```python
from build123d import *

# Parameters (mm, degrees)
F1_DEPTH = 50.8
F2_W     = 25.4
F2_H     = 15.645319
F3_DEPTH = 50.8
F4_W     = 21.66615
F4_H     = 13.618723
F5_DEPTH = 85.344


with BuildPart() as f1:
    # F0 (on Front) → F1 (new body)
    with BuildSketch(Plane.XZ):
        with BuildLine():
            Line((12.7, 38.1), (0, 38.1))
            Line((0, 38.1), (0, 0))
            Line((0, 0), (31.75, 0))
            Line((31.75, 0), (31.75, 12.7))
            ThreePointArc((31.75, 12.7), (19.301518, 23.207389), (12.7, 38.1))
        make_face()
    extrude(amount=F1_DEPTH)

    # F2 (on Right) → F3 (cut)
    with BuildSketch(Plane.YZ):
        with Locations((-24.754254, 30.332612)):
            Rectangle(F2_W, F2_H)
    extrude(amount=-F3_DEPTH, mode=Mode.SUBTRACT)

    # F4 (on Right) → F5 (cut)
    with BuildSketch(Plane.YZ):
        with Locations((-24.142282, 31.725436)):
            Rectangle(F4_W, F4_H)
    extrude(amount=F5_DEPTH, mode=Mode.SUBTRACT)


solid = f1.part
```
Can you work these out from the model? Positions are in its coordinate system, mm. A direction names the side the tool comes from. Round coordinates to 2 decimals unless told otherwise and drop trailing zeros. Loops run counter-clockwise (first coordinate to the right, second up) from the corner with the lowest first, then second, coordinate; pieces in that order, holes last.
Item 1: Suppose I cut it at D-D, the plane x = 17. Write out the boundary of the cut face in (y, z).
Item 2: Which directions (+Z, -Z, +X, -X, +Y, -Y) give clear straight access to the entire face, cutting with the end or side of a thin tool? Please do faces 1 (the flat face through (7, -34.975, 31)), 2 (the cylindrical face through (21.792, -25.044, 20.233)).
Item 3: Suppose I cut it at A-A, the plane z = 27. Write out the boundary of the cut face in (x, y), then the cut area to 3 significant figures.
Item 4: Suppose I cut it at C-C, the plane y = -32. Write out the boundary of the cut face in (x, z).
Item 5: Suppose I cut it at B-B, the plane x = 10. Write out the boundary of the cut face in (y, z).
Item 6: Please list where these lines run through material, in increasing order: L1, parallel to Y at x = 12.5, z = 27; L2, parallel to Z at x = 9.5, y = -22; L3, parallel to Z at x = 20.5, y = -10.
Item 7: Will these pins go through, and if not, where does the flat tip stop? pin 1 Ø1 at (y, z) = (-6, 24) entering from +X; pin 2 Ø1.5 at (x, y) = (28.5, -26.5) entering from +Z; pin 3 Ø1 at (y, z) = (-36, 33.5) entering from +X; pin 4 Ø8 at (x, y) = (28, -26.5) entering from -Z.
Reported:
1. outline: (-50.8, 0) - (0, 0) - (0, 26.67) - (-13.31, 26.67) - (-13.31, 24.92) - (-34.98, 24.92) - (-34.98, 26.67) - (-50.8, 26.67) - close
2. face 1: +Z, +X, -X
2. face 2: +Z, +X, +Y, -Y
3. outline: (0, -50.8) - (16.81, -50.8) - (16.81, -34.98) - (0, -34.98) - close; (0, -13.31) - (16.81, -13.31) - (16.81, 0) - (0, 0) - close
3. area: 490 mm2
4. outline: (0, 0) - (31.75, 0) - (31.75, 12.7) arc R36.31 cw to (18.1, 24.92) - (0, 24.92) - close
5. outline: (-50.8, 0) - (0, 0) - (0, 38.1) - (-13.31, 38.1) - (-13.31, 24.92) - (-34.98, 24.92) - (-34.98, 38.1) - (-50.8, 38.1) - close
6. L1: y = -50.8 to -34.98, -13.31 to 0
6. L2: z = 0 to 24.92
6. L3: z = 0 to 21.69
7. pin 1: stops at x = 19.08
7. pin 2: stops at z = 15.09
7. pin 3: stops at x = 14.08
7. pin 4: stops at z = 0
